Autodesk Inventor part; units mm, degrees
ref_plane "YZ Plane" through (0, 0, 0) normal (1, 0, 0) x (0, 1, 0)
ref_plane "XZ Plane" through (0, 0, 0) normal (0, 1, 0) x (-1, 0, 0)
ref_plane "XY Plane" through (0, 0, 0) normal (0, 0, 1) x (1, 0, 0)
sketch "Sketch1" plane through (0, 0, 0) normal (0, 1, 0) x (-1, 0, 0)
  circle A0 centre (0, 0) radius 25
  circle A1 centre (0, 0) radius 12.7
  circle A2 centre (0, 0) radius 5.2
  dimension "d1" = 50
  dimension "d14" = 25.4
  dimension "d15" = 10.4
extrude "Extrusion1" add sketch "Sketch1" along normal blind 20 contours A0 | A1 | A2
extrude "Extrusion2" cut sketch "Sketch1" along normal blind 11.4 contours A1
extrude "Extrusion3" cut sketch "Sketch1" along normal blind 20 contours A2
chamfer "Chamfer2" distance 11.4 distance2 7.5 1 edges at (12.7, 11.4, 0) measured on face at (-12.5355, 7.6, -2.0372)
properties part number "3. ring"
Read the model definition and answer for the solid it produces. Units are mm, in the model's axes. Coordinates: 2 decimals unless noted, no trailing zeros. Loops run counter-clockwise (first coordinate to the right, second up) from the corner with the lowest first, then second, coordinate; pieces in that order, holes last. Notation, with made-up numbers: (45.25, -1) - (94.25, -1) arc R21 ccw to (94.25, 9) - close; hole circle Ø10 at (19, -19.75). An arc over 180 degrees is marked (long way). Answer in a Markdown table with one row per item.
Q1. Find section D-D on x = 18. Write down the section's boundary in (y, z), plus the area to 3 significant figures.
Here are the results:
| item | result |
|---|---|
| outline | (0, -17.35) - (20, -17.35) - (20, 17.35) - (0, 17.35) - close |
| area | 694 mm^2 |
Q2. Straight lines are drawn through the part: line 1 along Z through (x, y) = (0, 16.75); line 2 along Z through (x, y) = (8.5, 2); line 3 along X through (y, z) = (12.5, -2.5). For each, find the intervals that lie inside material, in ascending order. Write a range as [from, to].
Here are the results:
| item | result |
|---|---|
| line 1 | z = [-25, -5.2], [5.2, 25] |
| line 2 | z = [-23.51, -7.57], [7.57, 23.51] |
| line 3 | x = [-24.87, -4.56], [4.56, 24.87] |
Q3. Find section C-C on y = 15. Write down the section's boundary in (x, z), plus the area to 3 significant figures.
Here are the results:
| item | result |
|---|---|
| outline | circle Ø50 at (0, 0); hole circle Ø10.4 at (0, 0) |
| area | 1,880 mm^2 |
Q4. Given P1, Ø12, axis at x = 17, y = 8, coming from the +Z side; P2, Ø12, axis at x = -0.5, z = 0, coming from the +Y side; P3, Ø1, axis at x = 7.5, y = 15.5, coming from the -Z side; P4, Ø5, axis at x = 2.5, z = -2, coming from the -Y side, each flat-ended and moving along its own axis, determine where each tip first touches the part or whether it passes through.
Here are the results:
| item | result |
|---|---|
| P1 | stops at z = 22.45 |
| P2 | stops at y = 20 |
| P3 | stops at z = -24 |
| P4 | stops at y = 10.64 |
Q5. The mould has two halves that part along X. Classify faces 1 (the cylindrical face through (-23.846, 9.86, -7.509)), 2 (the conical face through (5.16, 9.42, 3.96)), 3 (the flat face through (11.5, 0, 5.9)): pulls with the +X half, pulls with the -X half, needs draft (parallel to the pull), parting line crosses it, or undercut.
Here are the results:
| item | result |
|---|---|
| face 1 | parting line crosses it |
| face 2 | undercut |
| face 3 | needs draft |
